```python
from build123d import *

# Parameters (mm, degrees)
SKETCH1_W            = 139.65
SKETCH1_H            = 10
BASE_FLANGE1_DEPTH   = 1.016
EDGE_FLANGE1_DEPTH   = 40
FILLET1_R            = 2
M5_CLEARANCE_HOLE1_D = 5.5


# Sheet-metal steps are written as plain solids
with BuildPart() as part:
    # Sketch1 → Base-Flange1 (new body)
    with BuildSketch(Plane(origin=(0, 0, 0), x_dir=(1, 0, 0), z_dir=(0, 1, 0))):
        with Locations((-57.025509978, 5)):
            Rectangle(SKETCH1_W, SKETCH1_H)
    extrude(amount=-BASE_FLANGE1_DEPTH)

    # Edge-Flange1 section (across the edge) → Edge-Flange1 (add)
    with BuildSketch(Plane(origin=(-77.025509978, 0, 1.016), x_dir=(0, 0, -1), z_dir=(1, 0, 0))):
        with BuildLine():
            Line((-1.016, 1.016), (-1.016, 5.94))
            Line((-1.016, 5.94), (0, 5.94))
            Line((0, 5.94), (0, 1.016))
            ThreePointArc((0, 1.016), (0.29757951, 0.29757951), (1.016, 0))
            Line((1.016, 0), (1.016, -1.016))
            ThreePointArc((1.016, -1.016), (-0.420840979, -0.420840979), (-1.016, 1.016))
        make_face()
    extrude(amount=EDGE_FLANGE1_DEPTH)

    # Fillet1
    fillet1_edges = [part.edges().sort_by_distance(p)[0] for p in [
        (-77.025509978, 5.94, 1.524),
        (-37.025509978, 5.94, 1.524),
        (-126.850509978, -0.508, -10),
        (12.799490022, -0.508, -10),
        (12.799490022, -0.508, 0),
        (-126.850509978, -0.508, 0),
    ]]
    fillet(fillet1_edges, radius=FILLET1_R)

    # M5 Clearance Hole1 (through all)
    with Locations(Plane(origin=(0, 0, 0), x_dir=(1, 0, 0), z_dir=(0, 1, 0))):
        with Locations((-120.350509978, 5), (6.299490022, 5)):
            Hole(M5_CLEARANCE_HOLE1_D / 2)


solid = part.part
```
Geometry check sheet. Reference: the model listing, model coordinates, mm. A direction names the side the tool comes from. Coordinates: 2 decimals unless noted, no trailing zeros. Write each loop counter-clockwise with the first axis right and the second up, starting at its lowest first coordinate (ties: lowest second). Pieces come first, ordered by that corner, then holes. Notation, with made-up numbers: M 6,-35 L 23,-35 A30 ccw 23,-6 Z; hole C -9.5,-17 d3. An arc over 180 degrees is marked long. Use one line per item in the form item = value. Start each with the question number.
1) Section check A-A on z = -5. Enter the section's corners in (x, y), and give its area (3 significant figures).
2) Section check B-B on x = -54. Enter the section's corners in (y, z).
3) Thickness scan on probe 1 along Y at (x, z) = (-12.5, -3); probe 2 along X at (y, z) = (2.5, 1.75); probe 3 along Z at (x, y) = (-72.5, 5). Record the ranges inside material, lowest first. Write a range as from..to.
4) Set-up check for faces 1 (the flat face through (-57, 4, 1.016)), 2 (the cylindrical face through (-122.974, -0.515, -5.826)): record each of +Z, -Z, +X, -X, +Y, -Y from which the full face is reachable in a straight line by a thin tool's end or side.
5) Go/stop test with flat-tipped pins: pin 1 Ø0.6 at (y, z) = (1, 1) entering from -X; pin 2 Ø0.8 at (x, y) = (-20.5, -0.5) entering from +Z; pin 3 Ø1.6 at (y, z) = (2, 1) entering from +X. Record where each tip stops, or that it passes through.
6) Release check for a two-part mould opening along X. For faces 3 (the flat face through (-58, 0, -5)), 4 (the cylindrical face through (3.76, -0.52, -3.95)) record: pulls with the +X half, pulls with the -X half, needs draft (parallel to the pull), parting line crosses it, or undercut.
Responses:
q1.outline = M -126.85,-1.02 L -123.1,-1.02 L -123.1,0 L -126.85,0 Z; M -117.6,-1.02 L 3.55,-1.02 L 3.55,0 L -117.6,0 Z; M 9.05,-1.02 L 12.8,-1.02 L 12.8,0 L 9.05,0 Z
q1.area = 131 mm2
q2.outline = M -1.02,-10 L 0,-10 L 0,0 A1.02 cw 1.02,1.02 L 5.94,1.02 L 5.94,2.03 L 1.02,2.03 A2.03 ccw -1.02,0 Z
q3.probe_1 = -1.02..0
q3.probe_2 = -77.03..-37.03
q3.probe_3 = 1.02..2.03
q4.face_1 = -Z, +X, -X, +Y
q4.face_2 = +Y, -Y
q5.pin_1 = -77.03
q5.pin_2 = 0
q5.pin_3 = -37.03
q6.face_3 = needs draft
q6.face_4 = undercut
